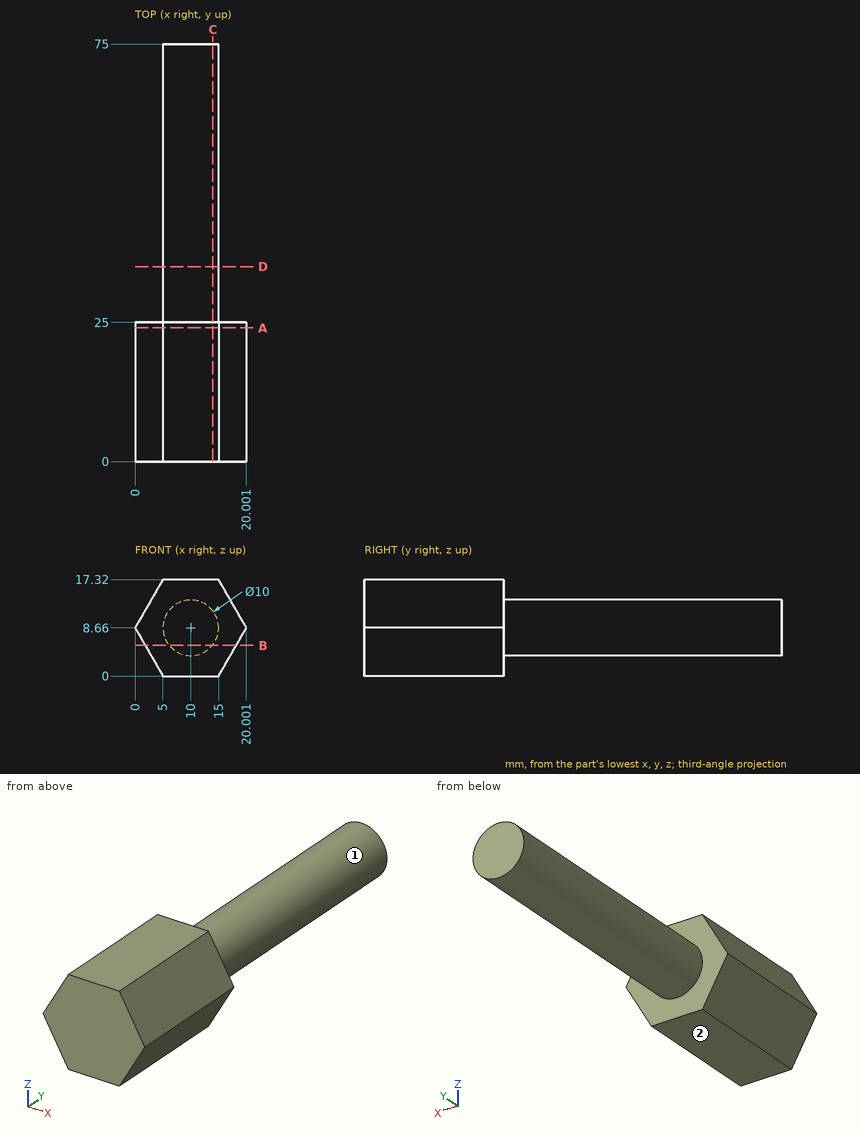
Study the drawing (mm; zero at the part's minimum x, y, z) and answer. A direction names the side the tool comes from. Give positions to 0.01 mm unless a question says otherwise; leave off trailing zeros. Loops run counter-clockwise (first coordinate to the right, second up) from the corner with the lowest first, then second, coordinate; pieces in that order, holes last. Notation, with made-up numbers: M -5.5,58 L 15.5,58 A17 ccw 15.5,81 Z; hole C 27.5,50.25 d5. An arc over 180 degrees is marked long. One line per item, written item: value.
1. Section C-C on x = 14 is taken. Determine the outline of the cut face in (y, z), plus the area to 3 significant figures.
Found:
outline: M 0,0 L 25,0 L 25,5.66 L 75,5.66 L 75,11.66 L 25,11.66 L 25,17.32 L 0,17.32 Z
area: 733 mm^2
2. Section B-B on z = 5.5 is taken. Determine the outline of the cut face in (x, y) (1 decimal), plus the area to 3 significant figures.
Found:
outline: M 1.8,0 L 18.2,0 L 18.2,25 L 13.9,25 L 13.9,75 L 6.1,75 L 6.1,25 L 1.8,25 Z
area: 796 mm^2
3. Section D-D on y = 35 is taken. Determine the outline of the cut face in (x, z).
Found:
outline: C 10,8.66 d10
4. Each of these flat-tipped pins is pushed along its axis until it touches: P1, Ø8, axis at x = 4, z = 4.5, coming from the +Y side; P2, Ø2, axis at x = 9, y = 51, coming from the +Z side; P3, Ø12, axis at x = 15.5, y = 38.5, coming from the -Z side; P4, Ø1.5, axis at x = 7.5, y = 50, coming from the -Z side. Where does it stop, or does it pass through?
Found:
P1: y = 75
P2: z = 13.66
P3: z = 3.66
P4: z = 3.98
5. Find the intervals of material crossed by probe 1 along Y at (x, z) = (8, 15.5); probe 2 along X at (y, z) = (8, 1.75); probe 3 along Z at (x, y) = (18.25, 8.5) (1 decimal), in increasing order.
Found:
probe 1: 0 to 25
probe 2: 3.99 to 16.01
probe 3: 5.6 to 11.7
6. Section A-A on y = 24 is taken. Determine the outline of the cut face in (x, z), plus the area to 3 significant figures.
Found:
outline: M 0,8.66 L 5,0 L 15,0 L 20,8.66 L 15,17.32 L 5,17.32 Z
area: 260 mm^2
7. For the marked faces 1 and 2, determine the directions among +Z, -Z, +X, -X, +Y, -Y from which every point of the face is accessible in a straight line to the end or side of a thin tool.
Found:
face 1: +Y
face 2: -Z, +X, -X, +Y, -Y
